from build123d import *

# Parameters (mm, degrees)
SKETCH1_R           = 75
BOSS_EXTRUDE1_DEPTH = 5
BOSS_EXTRUDE2_DEPTH = 5
BOSS_EXTRUDE3_START = -5
BOSS_EXTRUDE3_DEPTH = 5
SKETCH6_R           = 1.5
CUT_EXTRUDE1_DEPTH  = 5
SKETCH7_R           = 2.9
CUT_EXTRUDE2_DEPTH  = 2.5
SKETCH8_R           = 0.6
CUT_EXTRUDE3_DEPTH  = 5
CIRPATTERN1_COUNT   = 4
SKETCH10_R          = 1.25
CUT_EXTRUDE4_DEPTH  = 3
CIRPATTERN2_COUNT   = 4
SKETCH11_R          = 1.5
CUT_EXTRUDE5_DEPTH  = 5
SKETCH12_R          = 1.5
CUT_EXTRUDE6_DEPTH  = 5
CIRPATTERN3_COUNT   = 4
SKETCH13_R          = 2.488262112
CUT_EXTRUDE7_DEPTH  = 2.5
CIRPATTERN4_COUNT   = 4
SKETCH14_R          = 2.461092264
CUT_EXTRUDE8_DEPTH  = 2.5
SKETCH16_R          = 11.5
CUT_EXTRUDE10_DEPTH = 3


with BuildPart() as part:
    # Sketch1 → Boss-Extrude1 (new body)
    with BuildSketch(Plane(origin=(0, 0, 0), x_dir=(1, 0, 0), z_dir=(0, 1, 0))):
        with Locations(Location((0, 0, 0), (0, 0, 270))):
            Circle(SKETCH1_R)
    extrude(amount=BOSS_EXTRUDE1_DEPTH)

    # Sketch4 → Boss-Extrude2 (add)
    with BuildSketch(Plane.ZY.offset(25)):
        with BuildLine():
            Line((-13.582225242, 61.365780194), (-40, 5))
            Line((-40, 5), (40, 5))
            Line((40, 5), (13.582225242, 61.365780194))
            ThreePointArc((13.582225242, 61.365780194), (0, 70), (-13.582225242, 61.365780194))
        make_face()
    extrude(amount=BOSS_EXTRUDE2_DEPTH)

    # Sketch5 → Boss-Extrude3 (add)
    with BuildSketch(Plane.ZY.offset(-25).offset(BOSS_EXTRUDE3_START)):
        with BuildLine():
            Line((13.582225242, 61.365780194), (40, 5))
            Line((40, 5), (-40, 5))
            Line((-40, 5), (-13.582225242, 61.365780194))
            ThreePointArc((-13.582225242, 61.365780194), (0, 70), (13.582225242, 61.365780194))
        make_face()
    extrude(amount=BOSS_EXTRUDE3_DEPTH)

    # Sketch6 → Cut-Extrude1 (cut)
    with BuildSketch(Plane.ZY.offset(30)):
        with Locations((0, 55)):
            Circle(SKETCH6_R)
    extrude(amount=-CUT_EXTRUDE1_DEPTH, mode=Mode.SUBTRACT)

    # Sketch7 → Cut-Extrude2 (cut)
    with BuildSketch(Plane.ZY.offset(30)):
        with Locations((0, 55)):
            Circle(SKETCH7_R)
    extrude(amount=-CUT_EXTRUDE2_DEPTH, mode=Mode.SUBTRACT)

    # Sketch8 → Cut-Extrude3 (cut)
    with BuildSketch(Plane.ZY.offset(30)):
        with Locations((0, 62.25)):
            Circle(SKETCH8_R)
    cut_extrude3 = extrude(amount=-CUT_EXTRUDE3_DEPTH, mode=Mode.SUBTRACT)

    # CirPattern1: Cut-Extrude3 ×4 about axis
    cirpattern1_axis = Axis((0, 55, 0), (1, 0, 0))
    for i in range(1, CIRPATTERN1_COUNT):
        add(cut_extrude3.rotate(cirpattern1_axis, i * 360 / CIRPATTERN1_COUNT), mode=Mode.SUBTRACT)

    # Sketch10 → Cut-Extrude4 (cut)
    with BuildSketch(Plane.ZY.offset(30)):
        with Locations((0, 62.25)):
            Circle(SKETCH10_R)
    cut_extrude4 = extrude(amount=-CUT_EXTRUDE4_DEPTH, mode=Mode.SUBTRACT)

    # CirPattern2: Cut-Extrude4 ×4 about axis
    cirpattern2_axis = Axis((0, 55, 0), (1, 0, 0))
    for i in range(1, CIRPATTERN2_COUNT):
        add(cut_extrude4.rotate(cirpattern2_axis, i * 360 / CIRPATTERN2_COUNT), mode=Mode.SUBTRACT)

    # Sketch11 → Cut-Extrude5 (cut)
    with BuildSketch(Plane(origin=(0, 5, 0), x_dir=(1, 0, 0), z_dir=(0, 1, 0))):
        with Locations(Location((0, 0, 0), (0, 0, 270))):
            Circle(SKETCH11_R)
    extrude(amount=-CUT_EXTRUDE5_DEPTH, mode=Mode.SUBTRACT)

    # Sketch12 → Cut-Extrude6 (cut)
    with BuildSketch(Plane(origin=(0, 5, 0), x_dir=(1, 0, 0), z_dir=(0, 1, 0))):
        with Locations(Location((0, 12.5, 0), (0, 0, 270))):
            Circle(SKETCH12_R)
    cut_extrude6 = extrude(amount=-CUT_EXTRUDE6_DEPTH, mode=Mode.SUBTRACT)

    # CirPattern3: Cut-Extrude6 ×4 about axis
    cirpattern3_axis = Axis((0, 0, 0), (0, 1, 0))
    for i in range(1, CIRPATTERN3_COUNT):
        add(cut_extrude6.rotate(cirpattern3_axis, i * 360 / CIRPATTERN3_COUNT), mode=Mode.SUBTRACT)

    # Sketch13 → Cut-Extrude7 (cut)
    with BuildSketch(Plane(origin=(0, 5, 0), x_dir=(1, 0, 0), z_dir=(0, 1, 0))):
        with Locations(Location((0, 12.5, 0), (0, 0, 270))):
            Circle(SKETCH13_R)
    cut_extrude7 = extrude(amount=-CUT_EXTRUDE7_DEPTH, mode=Mode.SUBTRACT)

    # CirPattern4: Cut-Extrude7 ×4 about axis
    cirpattern4_axis = Axis((0, 0, 0), (0, 1, 0))
    for i in range(1, CIRPATTERN4_COUNT):
        add(cut_extrude7.rotate(cirpattern4_axis, i * 360 / CIRPATTERN4_COUNT), mode=Mode.SUBTRACT)

    # Sketch14 → Cut-Extrude8 (cut)
    with BuildSketch(Plane(origin=(0, 5, 0), x_dir=(1, 0, 0), z_dir=(0, 1, 0))):
        with Locations(Location((0, 0, 0), (0, 0, 270))):
            Circle(SKETCH14_R)
    extrude(amount=-CUT_EXTRUDE8_DEPTH, mode=Mode.SUBTRACT)

    # Sketch16 → Cut-Extrude10 (cut)
    with BuildSketch(Plane(origin=(-25, 0, 0), x_dir=(0, 0, -1), z_dir=(1, 0, 0))):
        with Locations((0, 55)):
            Circle(SKETCH16_R)
    extrude(amount=-CUT_EXTRUDE10_DEPTH, mode=Mode.SUBTRACT)


solid = part.part
The listing builds one solid part. Answer for the finished solid, in the listing's coordinates (mm). A direction names the side the tool comes from. Give positions to 0.01 mm unless a question says otherwise; leave off trailing zeros. Write each loop counter-clockwise with the first axis right and the second up, starting at its lowest first coordinate (ties: lowest second). Pieces come first, ordered by that corner, then holes. Notation, with made-up numbers: (30.25, 6) -> (64.25, 6) arc R28 cw to (64.25, 32) -> close; hole circle Ø11 at (-3, 52.5). An arc over 180 degrees is marked (long way). One line per question, with ' | ' between items. Start each with the question number.
1. Section D-D (x = 64.5) is taken. Determine the outline of the cut face in (y, z), plus the area to 3 significant figures.
2. Section C-C (y = 17.5) is taken. Determine the outline of the cut face in (x, z).
3. Given pin 1 Ø19.5 at (y, z) = (52.5, -11.5) entering from +X; pin 2 Ø1.5 at (x, z) = (-12, -0.5) entering from +Y; pin 3 Ø1.5 at (x, y) = (28.5, 40.5) entering from -Z; pin 4 Ø12 at (y, z) = (13, -6) entering from -X, each flat-ended and moving along its own axis, determine where each tip first touches the part or whether it passes through.
4. Section A-A (y = 33) is taken. Determine the outline of the cut face in (x, z).
5. Section B-B (z = -27) is taken. Determine the outline of the cut face in (x, y).
6. For faces 4 (the flat face through (-28, 52.6, -2.4)), 5 (the flat face through (-11, 2.5, 1)), 6 (the flat face through (27.535, 33.577, 26.606)), 7 (the flat face through (30, 31, 1)), 8 (the cylindrical face through (-27, 70, 0)), determine the directions among +Z, -Z, +X, -X, +Y, -Y from which every point of the face is accessible in a straight line to the end or side of a thin tool.
7. Find the intervals of material crossed by probe 1 along X at (y, z) = (33, -13); probe 2 along X at (y, z) = (57.5, 9); probe 3 along Y at (x, z) = (-45, 7), in increasing order.
8. For a pull along X with two mould halves and no side action, classify faces 1 (the flat face through (11, 2.5, -1)), 2 (the flat face through (-27.465, 33.577, -26.606)), 3 (the flat face through (-30, 31, -1)) as pulls with the +X half, pulls with the -X half, needs draft (parallel to the pull), parting line crosses it, or undercut.
Response values:
1) outline: (0, -38.27) -> (5, -38.27) -> (5, 38.27) -> (0, 38.27) -> close | area: 383 mm2
2) outline: (-30, -34.14) -> (-25, -34.14) -> (-25, 34.14) -> (-30, 34.14) -> close; (25, -34.14) -> (30, -34.14) -> (30, 34.14) -> (25, 34.14) -> close
3) pin 1: x = 30 | pin 2: through | pin 3: z = -23.71 | pin 4: x = -30
4) outline: (-30, -26.88) -> (-25, -26.88) -> (-25, 26.88) -> (-30, 26.88) -> close; (25, -26.88) -> (30, -26.88) -> (30, 26.88) -> (25, 26.88) -> close
5) outline: (-69.97, 0) -> (69.97, 0) -> (69.97, 5) -> (30, 5) -> (30, 32.74) -> (25, 32.74) -> (25, 5) -> (-25, 5) -> (-25, 32.74) -> (-30, 32.74) -> (-30, 5) -> (-69.97, 5) -> close
6) face 4: none | face 5: +Y | face 6: +Z, +X, -X, +Y | face 7: +Z, -Z, +X, +Y | face 8: +X, -X, +Y
7) probe 1: -30 to -25, 25 to 30 | probe 2: -30 to -28, 25 to 30 | probe 3: 0 to 5
8) face 1: undercut | face 2: needs draft | face 3: pulls with the -X half
